```python
from build123d import *

# Parameters (mm, degrees)
SKETCH1_W                         = 40
SKETCH1_H                         = 7.5
TAP_DRILL_FOR_M4_TAP1_D           = 3.3
TAP_DRILL_FOR_M4_TAP1_DEPTH       = 10
TAP_DRILL_FOR_M4_TAP1_CSINK_D     = 3.35
TAP_DRILL_FOR_M4_TAP1_CSINK_ANGLE = 90
TAP_DRILL_FOR_M4_TAP1_TIP         = 0.991420021
CUT_EXTRUDE1_DEPTH                = 13
CHAMFER1_SIZE                     = 0.6


with BuildPart() as part:
    # Sketch1 → Revolve1 (revolve)
    with BuildSketch(Plane.XY):
        with Locations((20, 3.75)):
            Rectangle(SKETCH1_W, SKETCH1_H)
    revolve(axis=Axis((40, 0, 0), (-1, 0, 0)))

    # Tap Drill for M4 Tap1
    with Locations(Plane(origin=(40, 0, 0), x_dir=(0, 0, -1), z_dir=(1, 0, 0))):
        with Locations((0, 0)):
            CounterSinkHole(TAP_DRILL_FOR_M4_TAP1_D / 2, TAP_DRILL_FOR_M4_TAP1_CSINK_D / 2, depth=TAP_DRILL_FOR_M4_TAP1_DEPTH, counter_sink_angle=TAP_DRILL_FOR_M4_TAP1_CSINK_ANGLE)
            with Locations((0, 0, -(TAP_DRILL_FOR_M4_TAP1_DEPTH + TAP_DRILL_FOR_M4_TAP1_TIP / 2))):  # 118° drill point
                Cone(0, TAP_DRILL_FOR_M4_TAP1_D / 2, TAP_DRILL_FOR_M4_TAP1_TIP, mode=Mode.SUBTRACT)

    # Sketch6 → Cut-Extrude1 (cut)
    with BuildSketch(Plane(origin=(40, 0, 0), x_dir=(0, 0, -1), z_dir=(1, 0, 0))):
        with BuildLine():
            Line((-6, -4.5), (-6, 4.5))
            ThreePointArc((-6, 4.5), (-7.5, 0), (-6, -4.5))
        make_face()
        with BuildLine():
            ThreePointArc((7.5, 0), (7.115124735, 2.371708245), (6, 4.5))
            Line((6, 4.5), (6, -4.5))
            ThreePointArc((6, -4.5), (7.115124735, -2.371708245), (7.5, 0))
        make_face()
    extrude(amount=-CUT_EXTRUDE1_DEPTH, mode=Mode.SUBTRACT)

    # Chamfer1
    chamfer1_edges = [part.edges().sort_by_distance(p)[0] for p in [
        (40, -7.5, 0),
        (40, 6.708203932, -3.354101966),
        (40, 0, 6),
        (40, 0, -6),
    ]]
    chamfer(chamfer1_edges, length=CHAMFER1_SIZE)


solid = part.part
```
Can you work these out from the model? Positions are in its coordinate system, mm. A direction names the side the tool comes from. Coordinates: 2 decimals unless noted, no trailing zeros. Order: outer loops, then holes, each group sorted by start corner. A loop starts at its lowest first (then second) coordinate and runs counter-clockwise, first axis right, second up.
1. I'm going to push flat-ended pins straight in: pin 1 (2 mm diameter, centred on x = 21.5, y = -5, fed in from -Z); pin 2 (2 mm diameter, centred on x = 15, z = 3, fed in from -Y); pin 3 (7 mm diameter, centred on x = 34.5, y = -0.5, fed in from -Z). Where does each tip first touch, or does it pass through?
2. For faces 5 (the face through (27, 0, -7)), 6 (the face through (27, 0, 7)), 7 (the face through (39.8, 7.1, 0.1)), which set-ups out of +Z, -Z, +X, -X, +Y, -Y let a thin tool reach every point of the face, with its end or its side?
3. If we section it at B-B (y = -2.5): Please give me the cut outline in (x, z).
4. If we section it at D-D (y = 3): Please give me the cut outline in (x, z).
5. If we section it at C-C (x = 4.5): Please give me the cut outline in (y, z).
6. Thinking about a two-plate mould opening in Z: for faces 1 (the face through (39.8, -7.1, -0.1)), 2 (the face through (33, 0, 6)), 3 (the face through (34.918, 1.115, -1.216)), 4 (the face through (29.2, -0.1, -0.3)), which applies, +Z half, -Z half, draft (parallel to the pull), parting line (faces both ways), or undercut?
7. I need wall thicknesses on line 1 (Z direction, x = 34.25, y = 0); line 2 (Y direction, x = 33, z = 0); line 3 (Z direction, x = 33.5, y = -0.75). Which ranges of each line are inside material? Lowest first, please.
8. If we section it at A-A (x = 37): Please give me the cut outline in (y, z), then the cut area to 3 significant figures.
Entries:
1. pin 1: stops at z = -6.34
1. pin 2: stops at y = -7.23
1. pin 3: stops at z = -6
2. face 5: -Z, +X, +Y, -Y
2. face 6: +Z, +X, +Y, -Y
2. face 7: +X, +Y
3. outline: (0, -7.07) - (27, -7.07) - (27, -6) - (39.4, -6) - (40, -5.4) - (40, 5.4) - (39.4, 6) - (27, 6) - (27, 7.07) - (0, 7.07) - close
4. outline: (0, -6.87) - (27, -6.87) - (27, -6) - (39.4, -6) - (40, -5.4) - (40, 5.4) - (39.4, 6) - (27, 6) - (27, 6.87) - (0, 6.87) - close
5. outline: circle Ø15 at (0, 0)
6. face 1: parting line
6. face 2: +Z half
6. face 3: undercut
6. face 4: undercut
7. line 1: z = -6 to -1.65, 1.65 to 6
7. line 2: y = -7.5 to -1.65, 1.65 to 7.5
7. line 3: z = -6 to -1.47, 1.47 to 6
8. outline: (-4.5, -6) - (4.5, -6) arc R7.5 ccw to (4.5, 6) - (-4.5, 6) arc R7.5 ccw to start; hole circle Ø3.3 at (0, 0)
8. area: 150 mm2
